CAD build for the part. Positions are in the model's coordinates, mm. A direction names the side the tool comes from. Coordinates: 2 decimals unless noted, no trailing zeros. Loops run counter-clockwise (first coordinate to the right, second up) from the corner with the lowest first, then second, coordinate; pieces in that order, holes last. Notation, with made-up numbers: (39, 79.25) -> (47, 79.25) arc R28 ccw to (47, 116.25) -> close; hole circle Ø10 at (14.25, -22). An arc over 180 degrees is marked (long way). Answer as CSV lines item,"result". Start each with the question number.
```python
from build123d import *

# Parameters (mm, degrees)
SKETCH_1_R      = 3.5
EXTRUDE_1_DEPTH = 2.5


with BuildPart() as part:
    # Эскиз1 → Бобышка-Вытянуть1 (new body)
    with BuildSketch(Plane.XY):
        Polygon((13, -13), (69.5, -13), (69.5, 13), (13, 13), (13, 32), (-13, 32), (-13, 13), (-69.5, 13), (-69.5, -13), (-13, -13), (-13, -32), (13, -32), align=None)
        with Locations((0, 24)):
            Circle(SKETCH_1_R, mode=Mode.SUBTRACT)
        with Locations((0, -24)):
            Circle(SKETCH_1_R, mode=Mode.SUBTRACT)
        with Locations((-61.5, 0)):
            Circle(SKETCH_1_R, mode=Mode.SUBTRACT)
        with Locations((-27.5, 0)):
            Circle(SKETCH_1_R, mode=Mode.SUBTRACT)
        with Locations(Location((27.5, 0, 0), (0, 0, 180))):  # turned: the seam where the file's is
            Circle(SKETCH_1_R, mode=Mode.SUBTRACT)
        with Locations(Location((61.5, 0, 0), (0, 0, 180))):  # turned: the seam where the file's is
            Circle(SKETCH_1_R, mode=Mode.SUBTRACT)
    extrude(amount=EXTRUDE_1_DEPTH)


solid = part.part
```
Q1. Saw through at A-A (y = 24). List the corners of the cut face in (x, z), and give its area (3 significant figures).
Q2. Saw through at D-D (y = 0). List the corners of the cut face in (x, z), and give its area (4 significant figures).
Q3. Which spindle directions (+Z, -Z, +X, -X, +Y, -Y) get a long thin tool onto all of the face, cutting with end or side? Do faces 1 (the flat face through (13, -23, 1)), 2 (the flat face through (-41, 13, 1)), 3 (the flat face through (-42, -13, 1)), 4 (the flat face through (13, 22, 1)). Say none if no direction does.
Q4. Pin check, flat tips, straight feed: pin 1 Ø1.5 at (y, z) = (15.5, 2) entering from +X; pin 2 Ø1.2 at (x, z) = (39.5, 1) entering from -Y; pin 3 Ø0.8 at (y, z) = (-18.5, 0.5) entering from -X. Stop position of each tip, or through.
Q5. Saw through at C-C (x = 0). List the corners of the cut face in (y, z), and give its area (3 significant figures).
Q6. Two-plate mould, pull along X, no slides. Class faces 5 (the cylindrical face through (-65, 0, 1)), 6 (the flat face through (-13, -22, 1)), 7 (the cylindrical face through (-0.46, -20.53, 1.23)), 8 (the flat face through (41, -13, 1)): pulls with the +X half, pulls with the -X half, needs draft (parallel to the pull), parting line crosses it, or undercut.
Q7. Probe probe 1 along Y at (x, z) = (0, 1.6); probe 2 along Y at (x, z) = (-27.5, 1.2); probe 3 along Y at (x, z) = (57.5, 1.05). List the from-to ranges inside material, lowest first. Write a range as from..to.
Q8. Saw through at B-B (z = 1.6). List the corners of the cut face in (x, y).
Ans:
1,outline,"(-13, 0) -> (-3.5, 0) -> (-3.5, 2.5) -> (-13, 2.5) -> close; (3.5, 0) -> (13, 0) -> (13, 2.5) -> (3.5, 2.5) -> close"
1,area,"47.5 mm²"
2,outline,"(-69.5, 0) -> (-65, 0) -> (-65, 2.5) -> (-69.5, 2.5) -> close; (-58, 0) -> (-31, 0) -> (-31, 2.5) -> (-58, 2.5) -> close; (-24, 0) -> (24, 0) -> (24, 2.5) -> (-24, 2.5) -> close; (31, 0) -> (58, 0) -> (58, 2.5) -> (31, 2.5) -> close; (65, 0) -> (69.5, 0) -> (69.5, 2.5) -> (65, 2.5) -> close"
2,area,"277.5 mm²"
3,face 1,"+Z, -Z, +X, -Y"
3,face 2,"+Z, -Z, -X, +Y"
3,face 3,"+Z, -Z, -X, -Y"
3,face 4,"+Z, -Z, +X, +Y"
4,pin 1,"stops at x = 13"
4,pin 2,"stops at y = -13"
4,pin 3,"stops at x = -13"
5,outline,"(-32, 0) -> (-27.5, 0) -> (-27.5, 2.5) -> (-32, 2.5) -> close; (-20.5, 0) -> (20.5, 0) -> (20.5, 2.5) -> (-20.5, 2.5) -> close; (27.5, 0) -> (32, 0) -> (32, 2.5) -> (27.5, 2.5) -> close"
5,area,"125 mm²"
6,face 5,"undercut"
6,face 6,"pulls with the -X half"
6,face 7,"undercut"
6,face 8,"needs draft"
7,probe 1,"y = -32..-27.5, -20.5..20.5, 27.5..32"
7,probe 2,"y = -13..-3.5, 3.5..13"
7,probe 3,"y = -13..13"
8,outline,"(-69.5, -13) -> (-13, -13) -> (-13, -32) -> (13, -32) -> (13, -13) -> (69.5, -13) -> (69.5, 13) -> (13, 13) -> (13, 32) -> (-13, 32) -> (-13, 13) -> (-69.5, 13) -> close; hole circle Ø7 at (-61.5, 0); hole circle Ø7 at (-27.5, 0); hole circle Ø7 at (0, -24); hole circle Ø7 at (0, 24); hole circle Ø7 at (27.5, 0); hole circle Ø7 at (61.5, 0)"
